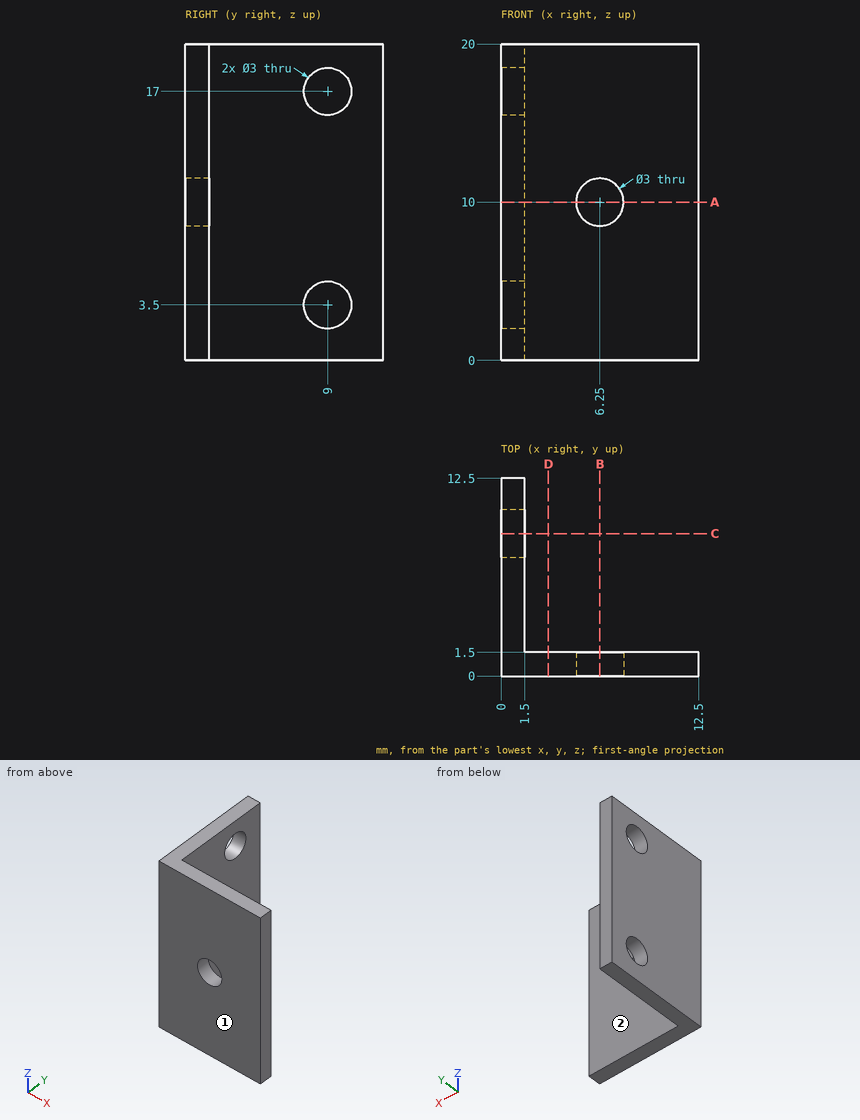
Geometry: see drawing. Coordinates: mm, zero at the bounding-box minimum. A direction names the side the tool comes from. Give positions to 0.01 mm unless a question says otherwise; leave off trailing zeros. Write each loop counter-clockwise with the first axis right and the second up, starting at its lowest first coordinate (ties: lowest second). Pieces come first, ordered by that corner, then holes. Notation, with made-up numbers: M 82.25,-18 L 96.25,-18 A22 ccw 96.25,17 Z; hole C 51.5,13 d1. An arc over 180 degrees is marked long. Answer as a JSON object with one key per item and string values.
Q1. Cut plane B-B, the plane x = 6.25. Return the cut outline in (y, z), then the cut area to 3 significant figures.
Geometry check:
{"outline": "M 0,0 L 1.5,0 L 1.5,8.5 L 0,8.5 Z; M 0,11.5 L 1.5,11.5 L 1.5,20 L 0,20 Z", "area": "25.5 mm^2"}
Q2. Access query for the marked faces 1 and 2. Directions: +Z, -Z, +X, -X, +Y, -Y. A direction counts if a zero-diameter tool reaches every point of the face in a straight line with its end or side. Return the directions, or none.
Geometry check:
{"face 1": "+Z, -Z, +X, -X, -Y", "face 2": "+Z, -Z, +X, +Y"}
Q3. Contact query for flat-ended pins moving along their axis: P1, Ø5.5, axis at x = 6, z = 11, coming from the +Y side; P2, Ø1.8, axis at x = 6.25, z = 10, coming from the +Y side; P3, Ø1.5, axis at y = 7.5, z = 12, coming from the -X side; P4, Ø3.5, axis at y = 8.5, z = 6, coming from the +X side. Output: stop coordinate, or through.
Geometry check:
{"P1": "stops at y = 1.5", "P2": "passes through", "P3": "stops at x = 0", "P4": "stops at x = 1.5"}
Q4. Cut plane A-A, the plane z = 10. Return the cut outline in (x, y).
Geometry check:
{"outline": "M 0,0 L 4.75,0 L 4.75,1.5 L 1.5,1.5 L 1.5,12.5 L 0,12.5 Z; M 7.75,0 L 12.5,0 L 12.5,1.5 L 7.75,1.5 Z"}
Q5. Cut plane D-D, the plane x = 3. Return the cut outline in (y, z).
Geometry check:
{"outline": "M 0,0 L 1.5,0 L 1.5,20 L 0,20 Z"}
Q6. Ray query, line 1 along Z through (x, y) = (0.85, 9); line 2 along X through (y, z) = (0.95, 10); line 3 along X through (y, z) = (8, 13.25). Return the intervals inside material, ascending.
Geometry check:
{"line 1": "z = 0 to 2, 5 to 15.5, 18.5 to 20", "line 2": "x = 0 to 4.75, 7.75 to 12.5", "line 3": "x = 0 to 1.5"}
Q7. Cut plane C-C, the plane y = 9. Return the cut outline in (x, z).
Geometry check:
{"outline": "M 0,0 L 1.5,0 L 1.5,2 L 0,2 Z; M 0,5 L 1.5,5 L 1.5,15.5 L 0,15.5 Z; M 0,18.5 L 1.5,18.5 L 1.5,20 L 0,20 Z"}
